Model file for the job. Use its own axes, mm. Face numbers are marked on the shaded views. Coordinates: 2 decimals unless noted, no trailing zeros. Write each loop counter-clockwise with the first axis right and the second up, starting at its lowest first coordinate (ties: lowest second). Pieces come first, ordered by that corner, then holes.
Q1. Drill centre lines: probe 1 along X at (y, z) = (1.1, 0); probe 2 along Y at (x, z) = (3, -3.75); probe 3 along Y at (x, z) = (-3, -1.75). Where is each one in solid material? Low to high.
Q2. Band-saw the part on C-C, the plane y = 8.5. Write the cut outline in (x, z) (3 decimals).
Q3. Pull direction X, two halves, no side cores. Call the marked faces 1, 2, 3 and 4: released by +X, released by -X, zero draft, split by the parting line, or undercut.
Q4. Band-saw the part on D-D, the plane x = 6. Write the cut outline in (y, z) (3 decimals).
Q5. Pin check, flat tips, straight feed: P1, Ø0.6, axis at x = -2.5, z = -1, coming from the +Y side; P2, Ø4, axis at x = 5, z = -3.5, coming from the +Y side; P3, Ø3, axis at x = -14, z = -3, coming from the +Y side; P4, Ø6, axis at x = -8.5, y = 20.5, coming from the +Z side. Stop position of each tip, or through.
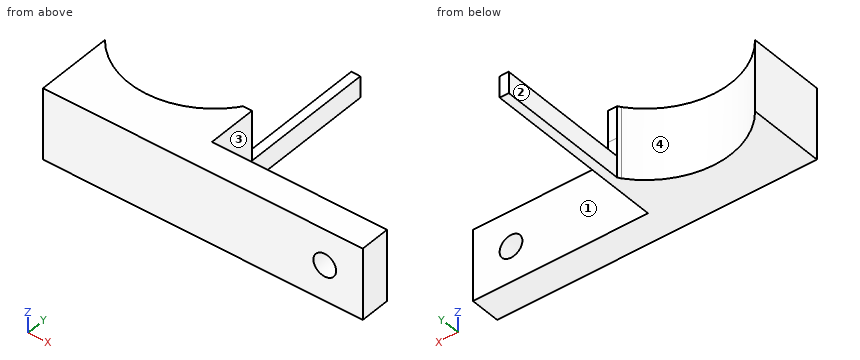
from build123d import *

# Parameters (mm, degrees)
SKETCH1_W           = 42.2
SKETCH1_H           = 9.41
BOSS_EXTRUDE1_DEPTH = 5.95
SKETCH2_W           = 23.1
SKETCH2_H           = 0.95
CUT_EXTRUDE1_DEPTH  = 10
SKETCH3_W           = 19.1
SKETCH3_H           = 9.41
BOSS_EXTRUDE2_DEPTH = 24.37
CUT_EXTRUDE8_DEPTH  = 20
SKETCH6_W           = 17.9
SKETCH6_H           = 9.41
CUT_EXTRUDE9_DEPTH  = 20.15
BOSS_EXTRUDE4_DEPTH = 9.41
SKETCH9_W           = 1.2
SKETCH9_H           = 4.2
CUT_EXTRUDE10_DEPTH = 19.74
SKETCH10_W          = 5.21
SKETCH10_H          = 1.92911269
CUT_EXTRUDE11_DEPTH = 19.74
SKETCH11_W          = 1.2
SKETCH11_H          = 2.39
CUT_EXTRUDE13_DEPTH = 17.810638
SKETCH12_W          = 9.41
SKETCH12_H          = 1.01654614
CUT_EXTRUDE14_DEPTH = 23.1
SKETCH13_R          = 1.5
CUT_EXTRUDE15_DEPTH = 23.1


with BuildPart() as part:
    # Sketch1 → Boss-Extrude1 (new body)
    with BuildSketch(Plane(origin=(0, 0, 0), x_dir=(1, 0, 0), z_dir=(0, 1, 0))):
        Rectangle(SKETCH1_W, SKETCH1_H)
    extrude(amount=BOSS_EXTRUDE1_DEPTH)

    # Sketch2 → Cut-Extrude1 (cut)
    with BuildSketch(Plane.XY.offset(4.705)):
        with Locations((9.55, 5.475)):
            Rectangle(SKETCH2_W, SKETCH2_H)
    extrude(amount=-CUT_EXTRUDE1_DEPTH, mode=Mode.SUBTRACT)

    # Sketch3 → Boss-Extrude2 (add)
    with BuildSketch(Plane(origin=(0, 5.95, 0), x_dir=(1, 0, 0), z_dir=(0, 1, 0))):
        with Locations((-11.55, 0)):
            Rectangle(SKETCH3_W, SKETCH3_H)
    extrude(amount=BOSS_EXTRUDE2_DEPTH)

    # Sketch5 → Cut-Extrude8 (cut)
    with BuildSketch(Plane(origin=(0, 0, -4.705), x_dir=(-1, 0, 0), z_dir=(0, 0, -1))):
        with BuildLine():
            Line((3.2, 10.501800084), (21.087895638, 10.16983908))
            ThreePointArc((21.087895638, 10.16983908), (12.062256205, 5.933823433), (3.2, 10.501800084))
        make_face()
    extrude(amount=-CUT_EXTRUDE8_DEPTH, mode=Mode.SUBTRACT)

    # Sketch6 → Cut-Extrude9 (cut)
    with BuildSketch(Plane(origin=(0, 30.32, 0), x_dir=(1, 0, 0), z_dir=(0, 1, 0))):
        with Locations((-12.15, 0)):
            Rectangle(SKETCH6_W, SKETCH6_H)
    extrude(amount=-CUT_EXTRUDE9_DEPTH, mode=Mode.SUBTRACT)

    # Sketch8 → Boss-Extrude4 (add)
    with BuildSketch(Plane.XY.offset(4.705)):
        Polygon((-3.455417816, 10.17), (-3.2, 10.580249423), (-3.2, 10.17), align=None)
    extrude(amount=-BOSS_EXTRUDE4_DEPTH)

    # Sketch9 → Cut-Extrude10 (cut)
    with BuildSketch(Plane(origin=(0, 30.32, 0), x_dir=(1, 0, 0), z_dir=(0, 1, 0))):
        with Locations((-2.6, -2.605)):
            Rectangle(SKETCH9_W, SKETCH9_H)
    extrude(amount=-CUT_EXTRUDE10_DEPTH, mode=Mode.SUBTRACT)

    # Sketch10 → Cut-Extrude11 (cut)
    with BuildSketch(Plane(origin=(-2, 0, 0), x_dir=(0, 0, -1), z_dir=(1, 0, 0))):
        with Locations((2.1, 29.355443655)):
            Rectangle(SKETCH10_W, SKETCH10_H)
    extrude(amount=-CUT_EXTRUDE11_DEPTH, mode=Mode.SUBTRACT)

    # Sketch11 → Cut-Extrude13 (cut)
    with BuildSketch(Plane(origin=(0, 28.39088731, 0), x_dir=(1, 0, 0), z_dir=(0, 1, 0))):
        with Locations((-2.6, 0.69)):
            Rectangle(SKETCH11_W, SKETCH11_H)
    extrude(amount=-CUT_EXTRUDE13_DEPTH, mode=Mode.SUBTRACT)

    # Sketch12 → Cut-Extrude14 (cut)
    with BuildSketch(Plane(origin=(21.1, 0, 0), x_dir=(0, 0, -1), z_dir=(1, 0, 0))):
        with Locations((0, 4.49172693)):
            Rectangle(SKETCH12_W, SKETCH12_H)
    extrude(amount=-CUT_EXTRUDE14_DEPTH, mode=Mode.SUBTRACT)

    # Sketch13 → Cut-Extrude15 (cut)
    with BuildSketch(Plane(origin=(0, 3.98345386, 0), x_dir=(1, 0, 0), z_dir=(0, 1, 0))):
        with Locations(Location((16.083417544, 0, 0), (0, 0, 270))):
            Circle(SKETCH13_R)
    extrude(amount=-CUT_EXTRUDE15_DEPTH, mode=Mode.SUBTRACT)


solid = part.part
Answer sheet:
1. probe 1: x = -21.1 to 14.58, 17.58 to 21.1
1. probe 2: y = 0 to 3.98
1. probe 3: y = 0 to 10.58
2. outline: (-21.1, -4.705) - (-19.44, -4.705) - (-19.44, 4.705) - (-21.1, 4.705) - close; (-5.103, -4.705) - (-2, -4.705) - (-2, 4.705) - (-5.103, 4.705) - close
3. face 1: zero draft
3. face 2: released by -X
3. face 3: released by +X
3. face 4: undercut
4. outline: (0, -4.705) - (3.983, -4.705) - (3.983, 4.705) - (0, 4.705) - close
5. P1: stops at y = 10.58
5. P2: stops at y = 3.98
5. P3: stops at y = 6.4
5. P4: passes through
